Can you work these out from the model? Positions are in its coordinate system, mm. A direction names the side the tool comes from. Give positions to 0.01 mm unless a question says otherwise; leave off trailing zeros. Order: outer loops, then holes, each group sorted by start corner. A loop starts at its lowest first (then second) coordinate and runs counter-clockwise, first axis right, second up. Notation, with made-up numbers: (22, 88) - (52, 88) arc R21 ccw to (52, 94) - close; hole circle Ø3 at (44.25, 3.5). An arc over 180 degrees is marked (long way). Answer as a JSON object with one key per item and string values.
Autodesk Inventor part; units mm, degrees
ref_plane "YZ Plane" through (0, 0, 0) normal (1, 0, 0) x (0, 1, 0)
ref_plane "XZ Plane" through (0, 0, 0) normal (0, 1, 0) x (-1, 0, 0)
ref_plane "XY Plane" through (0, 0, 0) normal (0, 0, 1) x (1, 0, 0)
sketch "Sketch1" plane through (0, 0, 0) normal (0, 0, 1) x (1, 0, 0)
  circle A0 centre (0, 0) radius 7.9375
  dimension "d0" = 15.875
extrude "Extrusion1" add sketch "Sketch1" along normal mid plane 90.4875
sketch "Sketch2" plane through (0, 0, 45.2437) normal (0, 0, 1) x (1, 0, 0)
  line L0 (-3.6662, 6.35) -> (3.6662, 6.35)
  line L1 (3.6662, 6.35) -> (7.3323, 0)
  line L2 (7.3323, 0) -> (3.6662, -6.35)
  line L3 (3.6662, -6.35) -> (-3.6662, -6.35)
  line L4 (-3.6662, -6.35) -> (-7.3323, 0)
  line L5 (-7.3323, 0) -> (-3.6662, 6.35)
  circle A0 centre (0, 0) radius 7.9375
  point P0 (0, -6.35)
  point P1 (0, 6.35)
  dimension "d3" = 12.7
extrude "Extrusion2" cut sketch "Sketch2" against normal blind 53.975
sketch "Sketch3" plane through (0, 0, 45.2437) normal (0, 0, 1) x (1, 0, 0)
  circle A0 centre (0, 0) radius 6.35
  circle A1 centre (0, 0) radius 7.9375
  line L0 (3.6662, 6.35) -> (-3.6662, 6.35)
  line L1 (7.3323, 0) -> (3.6662, 6.35)
  line L2 (3.6662, -6.35) -> (7.3323, 0)
  line L3 (-3.6662, -6.35) -> (3.6662, -6.35)
  line L4 (-7.3323, 0) -> (-3.6662, -6.35)
  line L5 (-3.6662, 6.35) -> (-7.3323, 0)
  point P0 (-5.4993, 3.175)
  point P1 (0, 6.35)
  point P2 (-5.4993, -3.175)
  point P3 (0, -6.35)
  point P4 (5.4993, -3.175)
  point P5 (5.4993, 3.175)
  dimension "d6" = 12.7
extrude "Extrusion3" cut sketch "Sketch3" against normal blind 6.35 contours A0 L1 L2 | A0 L0 L1 | L2 L3 A0 | A0 L5 L0 | L3 L4 A0 | A0 L4 L5
sketch "Sketch6" plane through (0, 0, 0) normal (1, 0, 0) x (0, 1, 0)
  line L0 (7.9375, -45.2437) -> (-7.9375, -45.2437) construction
  line L1 (-7.9375, -45.2437) -> (-7.9375, -8.7312) construction
  line L2 (-7.9375, -8.7312) -> (-6.35, -8.7312) construction
  line L3 (-6.35, -8.7312) -> (-6.35, 38.8938) construction
  line L4 (-6.35, 38.8938) -> (-6.35, 45.2437) construction
  line L5 (-6.35, 45.2437) -> (6.35, 45.2437) construction
  line L6 (6.35, 45.2437) -> (6.35, 38.8938) construction
  line L7 (6.35, 38.8938) -> (6.35, -8.7312) construction
  line L8 (6.35, -8.7312) -> (7.9375, -8.7312) construction
  line L9 (7.9375, -8.7312) -> (7.9375, -45.2437) construction
  line L10 (6.35, 45.2437) -> (-6.35, 45.2437)
  line L11 (-6.35, 45.2437) -> (-6.35, 38.8938)
  line L12 (-6.35, 38.8938) -> (6.35, 38.8938)
  line L13 (6.35, 38.8938) -> (6.35, 45.2437)
  line L14 (7.9375, -45.2437) -> (-7.9375, -45.2437) construction
  line L15 (-7.9375, -45.2437) -> (-7.9375, -8.7312) construction
  line L16 (-7.9375, -8.7312) -> (-6.35, -8.7312) construction
  line L17 (-6.35, -8.7312) -> (-6.35, 38.8938) construction
  line L18 (-6.35, 38.8938) -> (-6.35, 45.2437) construction
  line L19 (-6.35, 45.2437) -> (6.35, 45.2437) construction
  line L20 (6.35, 45.2437) -> (6.35, 38.8938) construction
  line L21 (6.35, 38.8938) -> (6.35, -8.7312) construction
  line L22 (6.35, -8.7312) -> (7.9375, -8.7312) construction
  line L23 (7.9375, -8.7312) -> (7.9375, -45.2437) construction
  line L24 (3.175, 38.8938) -> (6.35, 38.8938) construction
  line L25 (6.35, 38.8938) -> (-4.3066, 38.8938) construction
  line L26 (-3.175, 38.8938) -> (-6.35, 38.8938) construction
  line L27 (-7.9375, -45.2437) -> (-7.9375, -8.7312) construction
  line L28 (7.9375, -45.2437) -> (-7.9375, -45.2437)
  line L29 (-7.9375, -45.2437) -> (-7.9375, -41.6242)
  line L30 (-7.9375, -41.6242) -> (7.9375, -41.6242)
  line L31 (7.9375, -41.6242) -> (7.9375, -45.2437)
  point P0 (0, 0)
  dimension "d15" = 80.518
extrude "Extrusion6" cut sketch "Sketch6" along normal through all both and the other way through all
sketch "Sketch7" plane through (0, 0, -41.6242) normal (0, 0, -1) x (-1, 0, 0)
  circle A0 centre (0, 0) radius 6.35
  circle A1 centre (0, 0) radius 7.9375 construction
  circle A2 centre (0, 0) radius 7.9375
  circle A3 centre (0, 0) radius 7.9375 construction
  dimension "d18" = 12.7
extrude "Extrusion7" cut sketch "Sketch7" against normal blind 7.9375
properties part number "EL2-C2-003" material "Aluminum 6061"
Q1. I need wall thicknesses on L1, parallel to Y at x = 3.25, z = 16; L2, parallel to Z at x = 4.5, y = -4.75; L3, parallel to Z at x = -6.5, y = -3. Which ranges of each line are inside material? Lowest first, please.
Recorded:
{"L1": "y = -6.35 to 6.35", "L2": "z = -33.69 to 38.89", "L3": "z = -33.69 to -8.73"}
Q2. Which directions (+Z, -Z, +X, -X, +Y, -Y) give clear straight access to the entire face, cutting with the end or side of a thin tool? Please do faces 1 (the face through (0, 6.35, 15)), 2 (the face through (0, 7, -33.687)), 3 (the face through (-5.525, 3.131, 15.415)), 4 (the face through (5.474, 3.219, 15.415)), 5 (the face through (5.525, -3.131, 15.415)).
Recorded:
{"face 1": "+Z, +X, -X, +Y", "face 2": "-Z", "face 3": "+Z, -X, +Y", "face 4": "+Z, +X, +Y", "face 5": "+Z, +X, -Y"}
Q3. If we section it at D-D, the plane z = -27: Please give me the cut outline in (x, y) (1 decimal).
Recorded:
{"outline": "circle Ø15.9 at (0, 0)"}
Q4. If we section it at A-A, the plane z = 19.5: Please give me the cut outline in (x, y).
Recorded:
{"outline": "(-7.33, 0) - (-3.67, -6.35) - (3.67, -6.35) - (7.33, 0) - (3.67, 6.35) - (-3.67, 6.35) - close"}
Q5. If we section it at C-C, the plane x = -2.25: Please give me the cut outline in (y, z).
Recorded:
{"outline": "(-7.61, -33.69) - (-5.94, -33.69) - (-5.94, -41.62) - (5.94, -41.62) - (5.94, -33.69) - (7.61, -33.69) - (7.61, -8.73) - (6.35, -8.73) - (6.35, 38.89) - (-5.94, 38.89) - (-6.35, 38.89) - (-6.35, -8.73) - (-7.61, -8.73) - close"}
Q6. If we section it at B-B, the plane y = -4.75: Please give me the cut outline in (x, z).
Recorded:
{"outline": "(-6.36, -33.69) - (-4.21, -33.69) - (-4.21, -41.62) - (4.21, -41.62) - (4.21, -33.69) - (6.36, -33.69) - (6.36, -8.73) - (4.59, -8.73) - (4.59, 38.89) - (4.21, 38.89) - (-4.59, 38.89) - (-4.59, -8.73) - (-6.36, -8.73) - close"}
Q7. I'm going to push flat-ended pins straight in: pin 1 Ø1 at (x, z) = (-2.5, -9) entering from -Y; pin 2 Ø2 at (x, z) = (-1.5, 11) entering from -Y; pin 3 Ø4 at (x, z) = (-5, -25.5) entering from -Y. Where does each tip first touch, or does it pass through?
Recorded:
{"pin 1": "stops at y = -7.68", "pin 2": "stops at y = -6.35", "pin 3": "stops at y = -7.35"}
